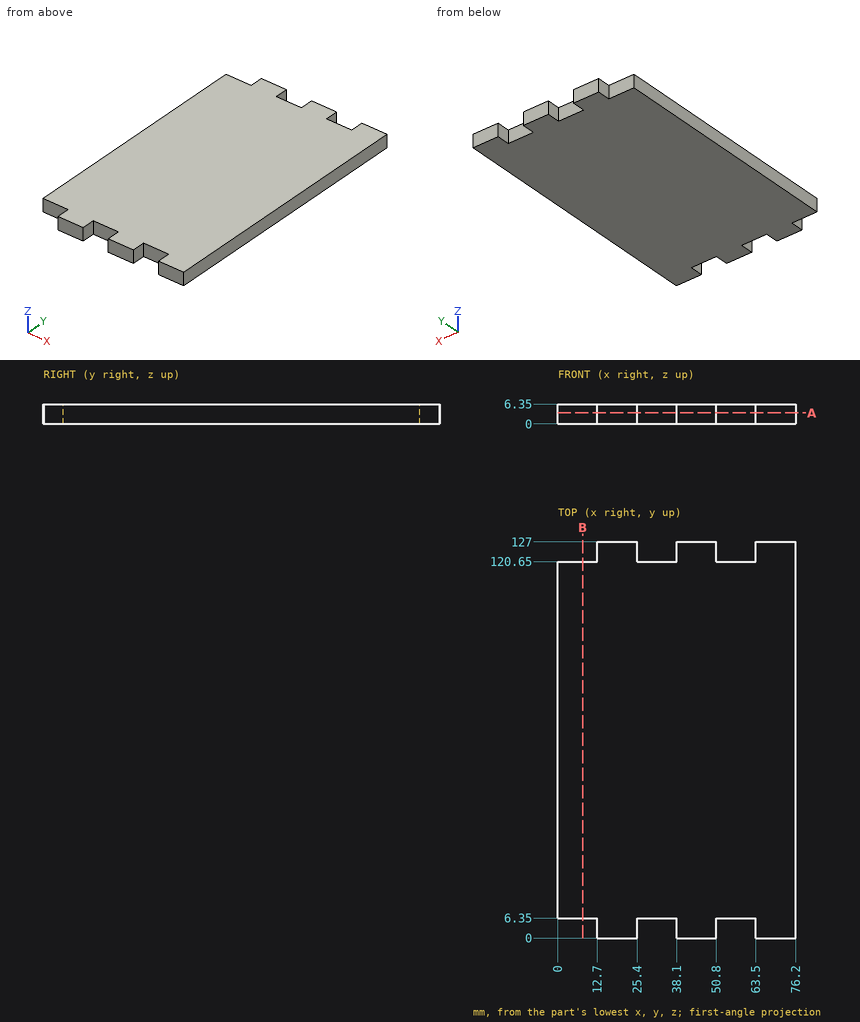
Design review of the part shown in the three views and the two pictorial views. Dimensions are in mm from the part's minimum x, y and z. Coordinates: 2 decimals unless noted, no trailing zeros. Order: outer loops, then holes, each group sorted by start corner. A loop starts at its lowest first (then second) coordinate and runs counter-clockwise, first axis right, second up.
1) Take a section at B-B, the plane x = 8. Give the boundary of the cut face in (y, z).
2) Clearance check with flat-ended pins moving along their axes: pin 1 (1.9 mm diameter, centred on y = 2.5, z = 4.5, fed in from -X); pin 2 (3 mm diameter, centred on x = 34, z = 4.5, fed in from +Y); pin 3 (3 mm diameter, centred on x = 34.5, z = 3.5, fed in from -Y). State where each tip first meets the part, or that it passes through.
3) Take a section at A-A, the plane z = 3.5. Give the boundary of the cut face in (x, y), and give its area (3 significant figures).
4) Wall thickness on line 1 along Y through (x, z) = (53.5, 5.75): over which ranges is the line inside the solid? List them lowest first.
Returned:
1. outline: (6.35, 0) - (120.65, 0) - (120.65, 6.35) - (6.35, 6.35) - close
2. pin 1: stops at x = 12.7
2. pin 2: stops at y = 120.65
2. pin 3: stops at y = 6.35
3. outline: (0, 6.35) - (12.7, 6.35) - (12.7, 0) - (25.4, 0) - (25.4, 6.35) - (38.1, 6.35) - (38.1, 0) - (50.8, 0) - (50.8, 6.35) - (63.5, 6.35) - (63.5, 0) - (76.2, 0) - (76.2, 127) - (63.5, 127) - (63.5, 120.65) - (50.8, 120.65) - (50.8, 127) - (38.1, 127) - (38.1, 120.65) - (25.4, 120.65) - (25.4, 127) - (12.7, 127) - (12.7, 120.65) - (0, 120.65) - close
3. area: 9,190 mm2
4. line 1: y = 6.35 to 120.65
